CAD build for the part. Positions are in the model's coordinates, mm. Face numbers are marked on the shaded views. Round coordinates to 2 decimals unless told otherwise and drop trailing zeros. Write each loop counter-clockwise with the first axis right and the second up, starting at its lowest first coordinate (ties: lowest second). Pieces come first, ordered by that corner, then holes. Notation, with made-up numbers: (59.5, -25) -> (98.5, -25) arc R4 cw to (98.5, -18) -> close; hole circle Ø3 at (-10.5, 30.5). An arc over 180 degrees is marked (long way). Answer in a Markdown table with one row per item. Add a question column.
```python
from build123d import *

# Parameters (mm, degrees)
REVOLVE7_ANGLE          = 180
SHELL1_T                = -2
CUT_EXTRUDE1_DEPTH      = 10
CUT_EXTRUDE2_DEPTH      = 123.474487139
CUT_EXTRUDE2_DEPTH_BACK = 123.474487139
CUT_EXTRUDE3_DEPTH      = 123.474487139
CUT_EXTRUDE3_DEPTH_BACK = 123.474487139
CUT_EXTRUDE10_DEPTH     = 150
BOSS_EXTRUDE1_DEPTH     = 1


with BuildPart() as part:
    # Sketch3 → Revolve7 (revolve)
    with BuildSketch(Plane(origin=(0, 0, 0), x_dir=(1, 0, 0), z_dir=(0, 1, 0))):
        with BuildLine():
            Line((0, 50), (0, -50))
            ThreePointArc((0, -50), (-50, 0), (0, 50))
        make_face()
    revolve(axis=Axis((0, 0, -50), (0, 0, 1)), revolution_arc=REVOLVE7_ANGLE)

    # Shell1
    shell1_openings = [part.faces().sort_by_distance(p)[0] for p in [
        (0, 0, 0),
    ]]
    offset(amount=SHELL1_T, openings=shell1_openings)

    # Sketch7 → Cut-Extrude1 (cut)
    with BuildSketch(Plane.XY.offset(50)):
        Polygon((-14.826397907, 0), (-3.370798864, -11.455599042), (15.645535913, 0), align=None)
    extrude(amount=-CUT_EXTRUDE1_DEPTH, mode=Mode.SUBTRACT)

    # Sketch9 → Cut-Extrude2 (cut, two sides: drawn at the far end of the back side and taken through both)
    with BuildSketch(Plane.XY.offset(50).offset(-CUT_EXTRUDE2_DEPTH_BACK)):
        Polygon((8.292044244, -4.429804855), (20.150794945, -10.787955598), (33.666572042, 0), (15.645535913, 0), align=None)
    extrude(amount=CUT_EXTRUDE2_DEPTH + CUT_EXTRUDE2_DEPTH_BACK, mode=Mode.SUBTRACT)

    # Sketch10 → Cut-Extrude3 (cut, two sides: drawn at the far end of the back side and taken through both)
    with BuildSketch(Plane.XY.offset(50).offset(-CUT_EXTRUDE3_DEPTH_BACK)):
        Polygon((-30.799589022, 0), (-43.496228113, 0), (-37.52885371, -5.967374403), align=None)
        Polygon((-14.826397907, 0), (-30.799589022, 0), (-25.323697422, -5.475891599), (-22.116726159, -2.268920336), (-17.177232044, -5.475891599), align=None)
    extrude(amount=CUT_EXTRUDE3_DEPTH + CUT_EXTRUDE3_DEPTH_BACK, mode=Mode.SUBTRACT)

    # Sketch12 → Cut-Extrude10 (cut)
    with BuildSketch(Plane(origin=(50, 0, 0), x_dir=(0, 0, -1), z_dir=(1, 0, 0))):
        Polygon((16.603317185, -8.277154343), (20.753512458, 0), (-28.80470168, 0), (2.281074676, -8.277154343), (8.384303018, -1.767044111), align=None)
    extrude(amount=-CUT_EXTRUDE10_DEPTH, mode=Mode.SUBTRACT)

    # Split1
    split(bisect_by=Plane(origin=(26.748894099, 0, 0), x_dir=(0, 0, 1), z_dir=(1, 0, 0)), keep=Keep.BOTTOM)

    # Sketch15 → Boss-Extrude1 (add)
    with BuildSketch(Plane(origin=(26.748894099, 0, 0), x_dir=(0, 0, -1), z_dir=(1, 0, 0))):
        with BuildLine():
            Line((-41.880896681, -5.521517702), (41.880896681, -5.521517702))
            ThreePointArc((41.880896681, -5.521517702), (0, -42.243303191), (-41.880896681, -5.521517702))
        make_face()
    extrude(amount=BOSS_EXTRUDE1_DEPTH)


solid = part.part
```
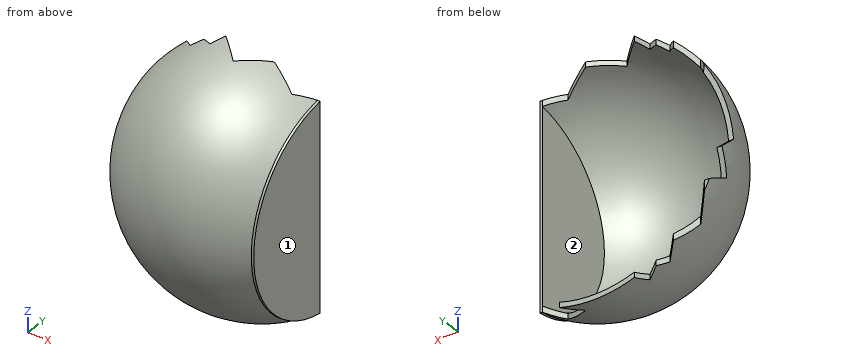
Item 1: Saw through at B-B on z = -6. Give the cut face in (x, y), then the cut area to 3 significant figures.
Item 2: Pin check, flat tips, straight feed: pin 1 (17 mm diameter, centred on y = -29, z = 4, fed in from -X); pin 2 (1 mm diameter, centred on x = 3, z = -26, fed in from -Y); pin 3 (4 mm diameter, centred on x = -21, z = 27.5, fed in from -Y). Stop position of each tip, or through.
Item 3: Drill centre lines: probe 1 along Z at (x, y) = (-34, -27); probe 2 along Z at (x, y) = (4.5, -8); probe 3 along X at (y, z) = (-6.5, -36). Where is each one in solid material? Low to high.
Item 4: Two-plate mould, pull along X, no slides. Class the marked faces 1 and 2: +X half, -X half, draft (parallel to the pull), parting line (faces both ways), or undercut.
Item 5: Saw through at C-C on y = -37. Give the cut face in (x, z), then the cut area to 3 significant figures.
Recorded:
| question | item | result |
|---|---|---|
| 1 | outline | (-49.45, -4.31) arc R49.64 ccw to (26.75, -41.82) -> (27.75, -41.82) -> (27.75, -5.52) -> (26.75, -5.52) -> (26.75, -39.4) arc R47.62 cw to (-47.43, -4.31) -> close |
| 1 | area | 239 mm2 |
| 2 | pin 1 | x = -45.48 |
| 2 | pin 2 | y = -42.91 |
| 2 | pin 3 | y = -37.91 |
| 3 | probe 1 | -24.8 to -20.47, 20.47 to 24.8 |
| 3 | probe 2 | -49.15 to -47.11, 47.11 to 49.15 |
| 3 | probe 3 | -34.08 to -31.08, 26.75 to 27.75 |
| 4 | face 1 | +X half |
| 4 | face 2 | undercut |
| 5 | outline | (26.75, -20.38) -> (27.75, -20.38) -> (27.75, 20.38) -> (26.75, 20.38) arc R33.63 ccw (long way) to start; hole (26.75, -14.82) -> (26.75, 14.82) arc R30.58 ccw (long way) to start |
| 5 | area | 542 mm2 |
